```python
from build123d import *

# Parameters (mm, degrees)
SKETCH1_R           = 5
SKETCH1_R_2         = 5.873519116
SKETCH1_R_3         = 2.75
BOSS_EXTRUDE1_DEPTH = 2.5


with BuildPart() as part:
    # Sketch1 → Boss-Extrude1 (new, symmetric)
    with BuildSketch(Plane.XY):
        with BuildLine():
            Line((-20.449003688, 0), (20.449003688, 0))
            ThreePointArc((20.449003688, 0), (26.876879785, 2.339555569), (30.297081218, 8.263518223))
            Line((30.297081218, 8.263518223), (47.929779289, 108.263518223))
            ThreePointArc((47.929779289, 108.263518223), (45.74214619, 116.427876097), (38.081701759, 120))
            Line((38.081701759, 120), (-38.081701759, 120))
            ThreePointArc((-38.081701759, 120), (-45.74214619, 116.427876097), (-47.929779289, 108.263518223))
            Line((-47.929779289, 108.263518223), (-30.297081218, 8.263518223))
            ThreePointArc((-30.297081218, 8.263518223), (-26.876879785, 2.339555569), (-20.449003688, 0))
        make_face()
        with Locations((28, 65)):
            Circle(SKETCH1_R, mode=Mode.SUBTRACT)
        with Locations((18, 20)):
            Circle(SKETCH1_R_2, mode=Mode.SUBTRACT)
        with Locations((0, 10)):
            Circle(SKETCH1_R_3, mode=Mode.SUBTRACT)
        with Locations((35, 110)):
            Circle(SKETCH1_R_3, mode=Mode.SUBTRACT)
        with Locations(Location((-18, 20, 0), (0, 0, 180))):
            Circle(SKETCH1_R_2, mode=Mode.SUBTRACT)
        with Locations(Location((-28, 65, 0), (0, 0, 180))):
            Circle(SKETCH1_R, mode=Mode.SUBTRACT)
        with Locations(Location((-35, 110, 0), (0, 0, 180))):
            Circle(SKETCH1_R_3, mode=Mode.SUBTRACT)
    extrude(amount=BOSS_EXTRUDE1_DEPTH, both=True)


solid = part.part
```
Here's how the part is built. I have some questions about the finished solid (model axes, mm). Give positions to 0.01 mm unless a question says otherwise; leave off trailing zeros. Loops run counter-clockwise (first coordinate to the right, second up) from the corner with the lowest first, then second, coordinate; pieces in that order, holes last. Notation, with made-up numbers: M 33.25,75 L 70.25,75 A24 cw 70.25,109 Z; hole C 1.25,82 d6. An arc over 180 degrees is marked long. Return JSON: item names as keys, results as strings.
Item 1: Please list where these lines run through material, in increasing order: line 1 (Y direction, x = -18, z = 1.15); line 2 (Y direction, x = 0, z = 0.5); line 3 (X direction, y = 64.5, z = 0.6).
A:
{"line 1": "y = 0 to 14.13, 25.87 to 120", "line 2": "y = 0 to 7.25, 12.75 to 120", "line 3": "x = -40.21 to -32.97, -23.03 to 23.03, 32.97 to 40.21"}
Item 2: Thinking about a two-plate mould opening in Y: for faces 1 (the flat face through (1, 120, 0)), 2 (the flat face through (38.99, 57.56, 0.04)), 3 (the cylindrical face through (16.727, 14.266, -0.035)), which applies, released by +Y, released by -Y, zero draft, split by the parting line, or undercut?
A:
{"face 1": "released by +Y", "face 2": "released by -Y", "face 3": "undercut"}
Item 3: Imagine slicing it at A-A on y = 110. List the corners of the cut face in (x, z) for me.
A:
{"outline": "M -48.08,-2.5 L -37.75,-2.5 L -37.75,2.5 L -48.08,2.5 Z; M -32.25,-2.5 L 32.25,-2.5 L 32.25,2.5 L -32.25,2.5 Z; M 37.75,-2.5 L 48.08,-2.5 L 48.08,2.5 L 37.75,2.5 Z"}
Item 4: Imagine slicing it at B-B on x = -18. List the corners of the cut face in (y, z) for me, then the cut area to 3 significant figures.
A:
{"outline": "M 0,-2.5 L 14.13,-2.5 L 14.13,2.5 L 0,2.5 Z; M 25.87,-2.5 L 120,-2.5 L 120,2.5 L 25.87,2.5 Z", "area": "541 mm^2"}
Item 5: I'm going to push flat-ended pins straight in: pin 1 Ø3 at (y, z) = (87, -0.5) entering from -X; pin 2 Ø10.5 at (x, y) = (18, 20) entering from -Z; pin 3 Ø3 at (y, z) = (47.5, 1) entering from +X; pin 4 Ø1 at (y, z) = (22, -1.5) entering from +X. Where does each tip first touch, or does it pass through?
A:
{"pin 1": "stops at x = -44.44", "pin 2": "passes through", "pin 3": "stops at x = 37.48", "pin 4": "stops at x = 32.81"}
Item 6: Imagine slicing it at D-D on y = 10. List the corners of the cut face in (x, z) for me.
A:
{"outline": "M -30.6,-2.5 L -2.75,-2.5 L -2.75,2.5 L -30.6,2.5 Z; M 2.75,-2.5 L 30.6,-2.5 L 30.6,2.5 L 2.75,2.5 Z"}
Item 7: Imagine slicing it at C-C on z = 1.4. List the corners of the cut face in (x, y) for me, then the cut area to 3 significant figures.
A:
{"outline": "M -47.93,108.26 L -30.3,8.26 A10 ccw -20.45,0 L 20.45,0 A10 ccw 30.3,8.26 L 47.93,108.26 A10 ccw 38.08,120 L -38.08,120 A10 ccw Z; hole C -35,110 d5.5; hole C -28,65 d10; hole C -18,20 d11.75; hole C 0,10 d5.5; hole C 18,20 d11.75; hole C 28,65 d10; hole C 35,110 d5.5", "area": "8,920 mm^2"}
